from build123d import *

# Parameters (mm, degrees)
SKETCH_W        = 212
SKETCH_H        = 146
PAD_DEPTH       = 20
SKETCH001_R     = 7.5
PAD001_DEPTH    = 15
SKETCH002_R     = 7.5
PAD002_DEPTH    = 15
CHAMFER_SIZE    = 2
CHAMFER001_SIZE = 2
CHAMFER002_SIZE = 8
SKETCH003_W     = 26
SKETCH003_H     = 14
POCKET_DEPTH    = 50
SKETCH004_W     = 100
SKETCH004_H     = 76
POCKET001_DEPTH = 15
CHAMFER003_SIZE = 1
CHAMFER004_SIZE = 1
SKETCH005_R     = 4.25
PAD003_DEPTH    = 10


with BuildPart() as part:
    # Sketch → Pad (new body)
    with BuildSketch(Plane.XY):
        with Locations((106, -73)):
            Rectangle(SKETCH_W, SKETCH_H)
    extrude(amount=PAD_DEPTH)

    # Sketch001 (on Face2 of Pad) → Pad001 (join)
    with BuildSketch(Plane.XZ.offset(146)):
        with Locations((197, 10)):
            Circle(SKETCH001_R)
    extrude(amount=PAD001_DEPTH)

    # Sketch002 (on Face2 of Pad001) → Pad002 (join)
    with BuildSketch(Plane(origin=(0, 0, 0), x_dir=(-1, 0, 0), z_dir=(0, 1, 0))):
        with Locations((-197, 10)):
            Circle(SKETCH002_R)
    extrude(amount=PAD002_DEPTH)

    # Chamfer
    chamfer_edges = [part.edges().sort_by_distance(p)[0] for p in [
        (204.5, 15, 10),
    ]]
    chamfer(chamfer_edges, length=CHAMFER_SIZE)

    # Chamfer001
    chamfer001_edges = [part.edges().sort_by_distance(p)[0] for p in [
        (189.5, -161, 10),
    ]]
    chamfer(chamfer001_edges, length=CHAMFER001_SIZE)

    # Chamfer002
    chamfer002_edges = [part.edges().sort_by_distance(p)[0] for p in [
        (212, -73, 0),
    ]]
    chamfer(chamfer002_edges, length=CHAMFER002_SIZE)

    # Sketch003 (on Face4 of Chamfer002) → Pocket (cut)
    with BuildSketch(Plane(origin=(0, 0, 0), x_dir=(0, -1, 0), z_dir=(-1, 0, 0))):
        with Locations((73, 10)):
            Rectangle(SKETCH003_W, SKETCH003_H)
    extrude(amount=-POCKET_DEPTH, mode=Mode.SUBTRACT)

    # Sketch004 (on Face6 of Pocket) → Pocket001 (cut)
    with BuildSketch(Plane.XY.offset(20)):
        with Locations((70, -73)):
            Rectangle(SKETCH004_W, SKETCH004_H)
    extrude(amount=-POCKET001_DEPTH, mode=Mode.SUBTRACT)

    # Chamfer003
    chamfer003_edges = [part.edges().sort_by_distance(p)[0] for p in [
        (102, 0, 0),
    ]]
    chamfer(chamfer003_edges, length=CHAMFER003_SIZE)

    # Chamfer004
    chamfer004_edges = [part.edges().sort_by_distance(p)[0] for p in [
        (102, -146, 0),
    ]]
    chamfer(chamfer004_edges, length=CHAMFER004_SIZE)

    # Sketch005 (on Face20 of Chamfer004) → Pad003 (join)
    with BuildSketch(Plane.XY.offset(5)):
        with Locations((85, -73)):
            Circle(SKETCH005_R)
    extrude(amount=PAD003_DEPTH)


solid = part.part
Geometry check sheet. Reference: the model listing, model coordinates, mm. A direction names the side the tool comes from. Give positions to 0.01 mm unless a question says otherwise; leave off trailing zeros. Write each loop counter-clockwise with the first axis right and the second up, starting at its lowest first coordinate (ties: lowest second). Pieces come first, ordered by that corner, then holes. Notation, with made-up numbers: M 72,-3 L 112,-3 A36 cw 112,35 Z; hole C 24.5,82 d1. An arc over 180 degrees is marked long. Answer as CSV lines item,"result". Start each with the question number.
Q1. Material ranges on L1, parallel to Y at x = 118.5, z = 19; L2, parallel to X at y = -62, z = 18; L3, parallel to Y at x = 155, z = 2.75, recorded low to high.
Q2. Release check for a two-part mould opening along Y. For faces 1 (the face through (105, 0, 10)), 2 (the face through (212, -74, 14)), 3 (the face through (85, -73, 15)) record: pulls with the +Y half, pulls with the -Y half, needs draft (parallel to the pull), parting line crosses it, or undercut.
Q3. Go/stop test with flat-tipped pins: pin 1 (4.5 mm diameter, centred on x = 69, z = 11.5, fed in from -Y); pin 2 (12 mm diameter, centred on x = 84, z = 15.5, fed in from +Y); pin 3 (3 mm diameter, centred on y = -53, z = 4, fed in from -X); pin 4 (4 mm diameter, centred on x = 86.5, y = -73, fed in from +Z). Record where each tip stops, or that it passes through.
Q4. Section check B-B, the plane x = 125.5. Record the cut outline in (y, z).
Q5. Section check C-C, the plane y = -46. Record the cut outline in (x, z).
Q6. Section check D-D, the plane x = 85. Record the cut outline in (y, z), then the cut area to 3 significant figures.
Q7. Section check A-A, the plane y = -73. Record the cut outline in (x, z), then the cut area to 3 significant figures.
Q8. Tool access check on faces 4 (the face through (14, -60, 10)), 5 (the face through (197, 15, 10)), 6 (the face through (84.08, -77.15, 9.93)). Record the directions out of +Z, -Z, +X, -X, +Y, -Y that give a thin tool (end or side, any length) a straight path to the whole face; none if there is none.
Geometry says:
1,L1,"-146 to -111, -35 to 0"
1,L2,"0 to 20, 120 to 212"
1,L3,"-146 to 0"
2,face 1,"pulls with the +Y half"
2,face 2,"needs draft"
2,face 3,"undercut"
3,pin 1,"y = -146"
3,pin 2,"y = 0"
3,pin 3,"x = 0"
3,pin 4,"z = 15"
4,outline,"M -146,1 L -145,0 L -1,0 L 0,1 L 0,20 L -146,20 Z"
5,outline,"M 0,0 L 204,0 L 212,8 L 212,20 L 120,20 L 120,5 L 20,5 L 20,20 L 0,20 Z"
6,outline,"M -146,1 L -145,0 L -1,0 L 0,1 L 0,20 L -35,20 L -35,5 L -68.75,5 L -68.75,15 L -77.25,15 L -77.25,5 L -111,5 L -111,20 L -146,20 Z"
6,area,"1,860 mm^2"
7,outline,"M 0,0 L 204,0 L 212,8 L 212,20 L 120,20 L 120,5 L 89.25,5 L 89.25,15 L 80.75,15 L 80.75,5 L 50,5 L 50,3 L 0,3 Z; M 0,17 L 20,17 L 20,20 L 0,20 Z"
7,area,"2,450 mm^2"
8,face 4,"-X"
8,face 5,"+Z, -Z, +X, -X, +Y"
8,face 6,"+Z"
